Here's how the part is built. I have some questions about the finished solid (model axes, mm). Face numbers are marked on the shaded views. A direction names the side the tool comes from. Coordinates: 2 decimals unless noted, no trailing zeros. Loops run counter-clockwise (first coordinate to the right, second up) from the corner with the lowest first, then second, coordinate; pieces in that order, holes last. Notation, with made-up numbers: (-33, -38) -> (5, -38) arc R22 cw to (5, -29) -> close; hole circle Ø8 at (5, 53.25). An arc over 180 degrees is marked (long way). Answer as a JSON object with one key per item and string values. Group by question number.
Q1. I want a section at B-B on z = 54. Write out the boundary of the cut face in (x, y).
Q2. I'm going to push flat-ended pins straight in: pin 1 (0.8 mm diameter, centred on y = 2.5, z = -20.5, fed in from -X); pin 2 (1.2 mm diameter, centred on x = 15.5, z = 56, fed in from -Y); pin 3 (4.5 mm diameter, centred on x = 15.5, z = 56, fed in from +Y); pin 4 (1.5 mm diameter, centred on x = 11.5, z = -15, fed in from -Y). Where does each tip first touch, or does it pass through?
Q3. I want a section at A-A on y = 15. Write out the boundary of the cut face in (x, z).
Q4. Thinking about a two-plate mould opening in Z: for the marked faces 1, 2 and 3, which applies, released by +Z, released by -Z, zero draft, split by the parting line, or undercut?
Q5. I want a section at C-C on x = 15.75. Write out the boundary of the cut face in (y, z), then the cut area to 3 significant figures.
Q6. I need wall thicknesses on line 1 (X direction, y = -0.5, z = -25); line 2 (Y direction, x = 15.25, z = -8); line 3 (Z direction, x = 15.5, y = 10.5). Which ranges of each line are inside material? Lowest first, please.
Q7. On a 3-axis mill with a long thin cutter (end or side, diameter ignored), from which of +Z, -Z, +X, -X, +Y, -Y can I reach the whole of each face in a straight line? I mean the marked faces 4 and 5. Say none if no direction works.
Q8. I want a section at D-D on x = 7. Write out the boundary of the cut face in (y, z).
```python
from build123d import *

# Parameters (mm, degrees)
SKETCH1_W           = 4
SKETCH1_H           = 75
BOSS_EXTRUDE1_DEPTH = 30
SKETCH4_R           = 0.5
SKETCH4_R_2         = 11.3
BOSS_EXTRUDE2_DEPTH = 8
BOSS_EXTRUDE3_DEPTH = 4
FILLET1_R           = 10
SKETCH9_R           = 2.5
SKETCH9_R_2         = 5
CUT_EXTRUDE2_DEPTH  = 4


with BuildPart() as part:
    # Sketch1 → Boss-Extrude1 (new body)
    with BuildSketch(Plane(origin=(0, 0, 0), x_dir=(1, 0, 0), z_dir=(0, 1, 0))):
        with Locations((16, -6.5)):
            Rectangle(SKETCH1_W, SKETCH1_H)
    extrude(amount=BOSS_EXTRUDE1_DEPTH)

    # Sketch4 → Boss-Extrude2 (add)
    with BuildSketch(Plane.ZY.offset(-14)):
        with BuildLine():
            Line((-22.142135624, 25.606601718), (-20.226017285, 23.690483379))
            ThreePointArc((-20.226017285, 23.690483379), (-23, 15), (-20.226017285, 6.309516621))
            Line((-20.226017285, 6.309516621), (-22.142135624, 4.393398282))
            ThreePointArc((-22.142135624, 4.393398282), (-22.142135624, 0.857864376), (-18.606601718, 0.857864376))
            Line((-18.606601718, 0.857864376), (-16.690483379, 2.773982715))
            ThreePointArc((-16.690483379, 2.773982715), (-8, 0), (0.690483379, 2.773982715))
            Line((0.690483379, 2.773982715), (2.606601718, 0.857864376))
            ThreePointArc((2.606601718, 0.857864376), (6.142135624, 0.857864376), (6.142135624, 4.393398282))
            Line((6.142135624, 4.393398282), (4.226017285, 6.309516621))
            ThreePointArc((4.226017285, 6.309516621), (7, 15), (4.226017285, 23.690483379))
            Line((4.226017285, 23.690483379), (6.142135624, 25.606601718))
            ThreePointArc((6.142135624, 25.606601718), (6.142135624, 29.142135624), (2.606601718, 29.142135624))
            Line((2.606601718, 29.142135624), (0.690483379, 27.226017285))
            ThreePointArc((0.690483379, 27.226017285), (-8, 30), (-16.690483379, 27.226017285))
            Line((-16.690483379, 27.226017285), (-18.606601718, 29.142135624))
            ThreePointArc((-18.606601718, 29.142135624), (-22.142135624, 29.142135624), (-22.142135624, 25.606601718))
        make_face()
        with Locations(Location((-20.374368671, 27.374368671, 0), (0, 0, 180))):
            Circle(SKETCH4_R, mode=Mode.SUBTRACT)
        with Locations((-8, 15)):
            Circle(SKETCH4_R_2, mode=Mode.SUBTRACT)
        with Locations(Location((4.374368671, 27.374368671, 0), (0, 0, 180))):
            Circle(SKETCH4_R, mode=Mode.SUBTRACT)
        with Locations(Location((4.374368671, 2.625631329, 0), (0, 0, 180))):
            Circle(SKETCH4_R, mode=Mode.SUBTRACT)
        with Locations(Location((-20.374368671, 2.625631329, 0), (0, 0, 180))):
            Circle(SKETCH4_R, mode=Mode.SUBTRACT)
    extrude(amount=BOSS_EXTRUDE2_DEPTH)

    # Sketch5 → Boss-Extrude3 (add)
    with BuildSketch(Plane.ZY.offset(-14)):
        Polygon((-31, 0), (-23, -3), (7, -3), (44, 0), (64, 0), (64, 30), (44, 30), (7, 33), (-23, 33), (-31, 30), align=None)
    extrude(amount=-BOSS_EXTRUDE3_DEPTH)

    # Fillet1
    # the kernel refuses this fillet: 10 mm, written as the material it takes off along each edge
    with BuildSketch(Plane(origin=(-3.325011704, 30, -31), x_dir=(0, 0.3511234415883908, 0.9363291775690449), z_dir=(1, 0, 0))) as fillet1_piece_1:
        with BuildLine():
            CenterArc((FILLET1_R * 0.693000468165, FILLET1_R), FILLET1_R, 200.55604522, 69.44395478)
            Line((-FILLET1_R * 0.243328709404, FILLET1_R * 0.648876558412), (0, 0))
            Line((0, 0), (FILLET1_R * 0.693000468165, 0))
        make_face()
    extrude(amount=38.650023408, mode=Mode.SUBTRACT)
    with BuildSketch(Plane(origin=(-3.325011704, 0, -31), x_dir=(0, -0.3511234415883923, 0.9363291775690443), z_dir=(1, 0, 0))) as fillet1_piece_2:
        with BuildLine():
            CenterArc((FILLET1_R * 0.693000468165, -FILLET1_R), FILLET1_R, 90, 69.44395478)
            Line((-FILLET1_R * 0.243328709404, -FILLET1_R * 0.648876558412), (0, 0))
            Line((0, 0), (FILLET1_R * 0.693000468165, 0))
        make_face()
    extrude(amount=38.650023408, mode=Mode.SUBTRACT)
    with BuildSketch(Plane(origin=(12.988146779, 33, 7), x_dir=(0, -0.0808158687660647, 0.9967290481146751), z_dir=(1, 0, 0)), Plane(origin=(12.988146779, -3, 7), x_dir=(0, 0, -1), z_dir=(1, 0, 0))) as fillet1_piece_3:
        with BuildLine():
            CenterArc((FILLET1_R * 0.0404741288471, FILLET1_R), FILLET1_R, 265.364536573, 4.635463427)
            Line((-FILLET1_R * 0.040341739919, FILLET1_R * 0.00327095188532), (0, 0))
            Line((0, 0), (FILLET1_R * 0.0404741288471, 0))
        make_face()
    extrude(amount=6.023706442, mode=Mode.SUBTRACT)
    with BuildSketch(Plane(origin=(9.466635456, 33, -23), x_dir=(0, 0, 1), z_dir=(1, 0, 0)), Plane(origin=(9.466635456, -3, -23), x_dir=(0, 0.35112344158839215, -0.9363291775690443), z_dir=(1, 0, 0))) as fillet1_piece_4:
        with BuildLine():
            CenterArc((FILLET1_R * 0.181334581773, FILLET1_R), FILLET1_R, 249.44395478, 20.55604522)
            Line((-FILLET1_R * 0.169788859816, FILLET1_R * 0.063670822431), (0, 0))
            Line((0, 0), (FILLET1_R * 0.181334581773, 0))
        make_face()
    extrude(amount=13.066729089, mode=Mode.SUBTRACT)

    # Sketch9 → Cut-Extrude2 (cut)
    with BuildSketch(Plane.ZY.offset(-14)):
        with Locations((54, 15)):
            Circle(SKETCH9_R)
        with Locations((29, 15)):
            Circle(SKETCH9_R)
        with Locations((-8, 15)):
            Circle(SKETCH9_R_2)
    extrude(amount=-CUT_EXTRUDE2_DEPTH, mode=Mode.SUBTRACT)


solid = part.part
```
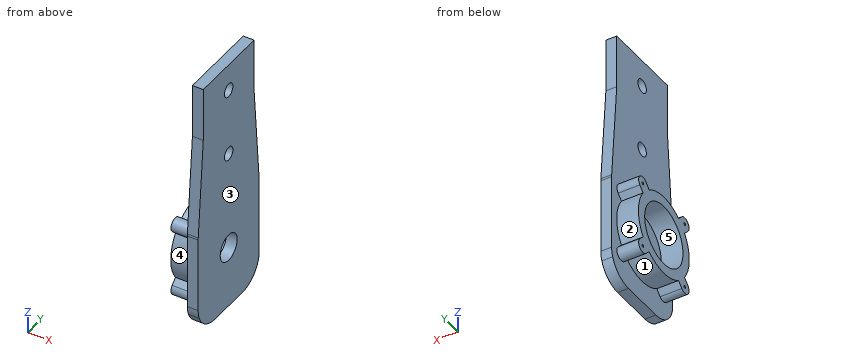
Result set:
{
 "1": {"outline": "(14, 0) -> (18, 0) -> (18, 12.5) -> (14, 12.5) -> close; (14, 17.5) -> (18, 17.5) -> (18, 30) -> (14, 30) -> close"},
 "2": {"pin 1": "stops at x = 6", "pin 2": "stops at y = 0", "pin 3": "stops at y = 30", "pin 4": "stops at y = 1.36"},
 "3": {"outline": "(6, -23) -> (14, -23) -> (14, -31) -> (18, -31) -> (18, -13) -> (14, -13) -> (14, -19.3) -> (6, -19.3) -> close; (6, 3.3) -> (14, 3.3) -> (14, -3) -> (18, -3) -> (18, 26.5) -> (14, 26.5) -> (14, 7) -> (6, 7) -> close; (14, 31.5) -> (18, 31.5) -> (18, 51.5) -> (14, 51.5) -> close; (14, 56.5) -> (18, 56.5) -> (18, 64) -> (14, 64) -> close"},
 "4": {"face 1": "released by -Z", "face 2": "undercut", "face 3": "zero draft"},
 "5": {"outline": "(-3, -21.19) arc R10 ccw to (-2.4, -24.6) arc R10 ccw to (6.93, -31) -> (23.07, -31) arc R10 ccw to (32.4, -24.6) arc R10 ccw to (33, -21.19) -> (33, 6.6) arc R10 ccw to (32.97, 7.4) -> (30, 44) -> (30, 64) -> (0, 64) -> (0, 44) -> (-2.97, 7.4) arc R10 ccw to (-3, 6.6) -> close; hole circle Ø10 at (15, -8); hole circle Ø5 at (15, 29); hole circle Ø5 at (15, 54)", "area": "3,030 mm²"},
 "6": {"line 1": "x = 14 to 18", "line 2": "y = -3 to 10, 20 to 33", "line 3": "z = -31 to -10.18, -5.82 to 64"},
 "7": {"face 4": "-X, -Y", "face 5": "-X"},
 "8": {"outline": "(0.86, -18.61) arc R2.5 ccw to (4.39, -22.14) -> (6.31, -20.23) arc R15 ccw to (23.69, -20.23) -> (25.61, -22.14) arc R2.5 ccw to (29.14, -18.61) -> (27.23, -16.69) arc R15 ccw to (27.23, 0.69) -> (29.14, 2.61) arc R2.5 ccw to (25.61, 6.14) -> (23.69, 4.23) arc R15 ccw to (6.31, 4.23) -> (4.39, 6.14) arc R2.5 ccw to (0.86, 2.61) -> (2.77, 0.69) arc R15 ccw to (2.77, -16.69) -> close; hole circle Ø1 at (2.63, -20.37); hole circle Ø1 at (2.63, 4.37); hole circle Ø22.6 at (15, -8); hole circle Ø1 at (27.37, -20.37); hole circle Ø1 at (27.37, 4.37)"}
}
